Part model, mm, in its own coordinate system. A direction names the side the tool comes from. Coordinates: 2 decimals unless noted, no trailing zeros. Loops run counter-clockwise (first coordinate to the right, second up) from the corner with the lowest first, then second, coordinate; pieces in that order, holes last. Notation, with made-up numbers: M -1.75,37.5 L 55.25,37.5 A34 ccw 55.25,73.5 Z; hole C 7.5,-29 d2. An arc over 180 degrees is marked long. Answer as CSV lines item,"result". Start each with the question number.
from build123d import *

# Parameters (mm, degrees)
BOSS_EXTRUDE1_DEPTH     = 3.175
FILLET1_R               = 0.254
CUT_EXTRUDE1_REACH      = 32.259
CUT_EXTRUDE2_DEPTH      = 29.575
CUT_EXTRUDE2_DEPTH_BACK = 29.575
SKETCH6_W               = 25.4
SKETCH6_H               = 1.5875


with BuildPart() as part:
    # Sketch1 → Boss-Extrude1 (new, symmetric)
    with BuildSketch(Plane(origin=(0, 0, 0), x_dir=(1, 0, 0), z_dir=(0, 1, 0))):
        Polygon((15.169114158, 0), (7.786246133, -3.645659373), (0.403378108, 0), (2.469114158, 0), (2.469114158, 25.4), (15.169114158, 25.4), align=None)
    extrude(amount=BOSS_EXTRUDE1_DEPTH, both=True)

    # Fillet1
    fillet1_edges = [part.edges().sort_by_distance(p)[0] for p in [
        (2.469114158, 0, 0),
        (15.169114158, 0, 0),
        (7.786246133, 0, 3.645659373),
        (0.403378108, 0, 0),
    ]]
    fillet(fillet1_edges, radius=FILLET1_R)

    # Sketch5 → Cut-Extrude1 (cut, up to next)
    with BuildSketch(Plane(origin=(0, 3.175, 0), x_dir=(1, 0, 0), z_dir=(0, 1, 0)), mode=Mode.PRIVATE) as cut_extrude1_sk1:
        with BuildLine():
            Line((11.409914158, 20.955), (11.409914158, 2.5908))
            ThreePointArc((11.409914158, 2.5908), (8.819114158, 0), (6.228314158, 2.5908))
            Line((6.228314158, 2.5908), (6.228314158, 20.955))
            ThreePointArc((6.228314158, 20.955), (8.819114158, 23.5458), (11.409914158, 20.955))
        make_face()
    cut_extrude1_tool1 = extrude(cut_extrude1_sk1.sketch, amount=-CUT_EXTRUDE1_REACH, mode=Mode.PRIVATE) & part.part
    add(cut_extrude1_tool1.solids().sort_by_distance((8.819114, 3.175, -11.7729))[0], mode=Mode.SUBTRACT)

    # Sketch6 → Cut-Extrude2 (cut, two sides: drawn at the far end of the back side and taken through both)
    with BuildSketch(Plane.ZY.offset(-2.469114158).offset(-CUT_EXTRUDE2_DEPTH_BACK)):
        with Locations((-12.7, 2.38125)):
            Rectangle(SKETCH6_W, SKETCH6_H)
        with Locations((-12.7, -2.38125)):
            Rectangle(SKETCH6_W, SKETCH6_H)
    extrude(amount=CUT_EXTRUDE2_DEPTH + CUT_EXTRUDE2_DEPTH_BACK, mode=Mode.SUBTRACT)


solid = part.part
Q1. Slice it at C-C, the plane x = 6.5. Write the cut outline in (y, z) (1 decimal).
Q2. Wall check: L1, parallel to X at y = -0.75, z = -20.25; L2, parallel to Y at x = 2.5, z = -12.5; L3, parallel to X at y = 0.75, z = -23. Give the ranges that are in metal, low to high.
Q3. Slice it at A-A, the plane y = -0.75. Write the cut outline in (x, z) (3 decimals), and give its area (3 significant figures).
Q4. Tool access for faces 5 (the face through (12, 1.588, -13)), 6 (the face through (12, -1.588, -13)), 7 (the face through (8.9, 0, 0)), 8 (the face through (8, -3.175, 1)): list every direction of +Z, -Z, +X, -X, +Y, -Y with a clear straight run to the whole face (end or side of a thin tool).
Q5. Slice it at B-B, the plane z = -14.75. Write the cut outline in (x, y), and give its area (3 significant figures).
Q6. Flat gauge pins, fed straight in: P1, Ø1.5, axis at y = 1, z = -4.5, coming from the -X side; P2, Ø1, axis at x = 4, z = -3.5, coming from the -Y side; P3, Ø4, axis at x = 6, z = -17.5, coming from the +Y side. Where does each tip first touch, or does it go through?
Q7. Slice it at D-D, the plane y = 2.5. Write the cut outline in (x, z), and give its area (3 significant figures).
Q8. Two-plate mould, pull along X, no slides. Class faces 1 (the face through (2.469, 0, -13)), 2 (the face through (6.228, 0, -12)), 3 (the face through (8.762, 0.022, -23.545)), 4 (the face through (15.169, 0, -13)): +X half, -X half, draft (parallel to the pull), parting line (faces both ways), or undercut.
Solved:
1,outline,"M -3.2,0 L -1.6,0 L -1.6,-1.4 L 1.6,-1.4 L 1.6,0 L 3.2,0 L 3.2,3 L -3.2,3 Z; M -1.6,-25.4 L 1.6,-25.4 L 1.6,-22.1 L -1.6,-22.1 Z"
2,L1,"x = 2.47 to 6.23, 11.41 to 15.17"
2,L2,"y = -1.59 to 1.59"
2,L3,"x = 2.47 to 7.23, 10.41 to 15.17"
3,outline,"M 1.379,0.482 A0.254 ccw 1.491,0 L 2.215,0 A0.254 cw 2.469,-0.254 L 2.469,-25.4 L 15.169,-25.4 L 15.169,-0.158 A0.254 ccw 15.028,0.07 L 7.899,3.59 A0.254 ccw 7.674,3.59 Z; hole M 6.228,-20.955 A2.591 ccw 11.41,-20.955 L 11.41,-2.591 A2.591 ccw 6.228,-2.591 Z"
3,area,"233 mm2"
4,face 5,"-Z, +X, -X, +Y"
4,face 6,"-Z, +X, -X, -Y"
4,face 7,"+Y, -Y"
4,face 8,"+Z, -Z, +X, -X, -Y"
5,outline,"M 2.47,-1.59 L 6.23,-1.59 L 6.23,1.59 L 2.47,1.59 Z; M 11.41,-1.59 L 15.17,-1.59 L 15.17,1.59 L 11.41,1.59 Z"
5,area,"23.9 mm2"
6,P1,"stops at x = 2.47"
6,P2,"stops at y = -1.59"
6,P3,"stops at y = 1.59"
7,outline,"M 1.38,0.48 A0.25 ccw 1.49,0 L 15.11,0 A0.25 ccw 15.03,0.07 L 7.9,3.59 A0.25 ccw 7.67,3.59 Z"
7,area,"26.7 mm2"
8,face 1,"-X half"
8,face 2,"undercut"
8,face 3,"undercut"
8,face 4,"+X half"
